from build123d import *

# Parameters (mm, degrees)
SKETCH2_W           = 150
SKETCH2_H           = 75
SKETCH2_W_2         = 25
SKETCH2_H_2         = 62.5
SKETCH2_W_3         = 15
SKETCH2_W_4         = 10
SKETCH2_W_5         = 5
SKETCH2_W_6         = 2.5
SKETCH2_W_7         = 1
BOSS_EXTRUDE1_DEPTH = 20


with BuildPart() as part:
    # Sketch2 → Boss-Extrude1 (new body)
    with BuildSketch(Plane(origin=(0, 0, 0), x_dir=(1, 0, 0), z_dir=(0, 1, 0))):
        with Locations((75, 37.5)):
            Rectangle(SKETCH2_W, SKETCH2_H)
        with Locations((21.5, 36.25)):
            Rectangle(SKETCH2_W_2, SKETCH2_H_2, mode=Mode.SUBTRACT)
        with Locations((66.5, 36.25)):
            Rectangle(SKETCH2_W_3, SKETCH2_H_2, mode=Mode.SUBTRACT)
        with Locations((94, 36.25)):
            Rectangle(SKETCH2_W_4, SKETCH2_H_2, mode=Mode.SUBTRACT)
        with Locations((111.5, 36.25)):
            Rectangle(SKETCH2_W_5, SKETCH2_H_2, mode=Mode.SUBTRACT)
        with Locations((122.75, 36.25)):
            Rectangle(SKETCH2_W_6, SKETCH2_H_2, mode=Mode.SUBTRACT)
        with Locations((127.5, 36.25)):
            Rectangle(SKETCH2_W_7, SKETCH2_H_2, mode=Mode.SUBTRACT)
    extrude(amount=BOSS_EXTRUDE1_DEPTH)


solid = part.part
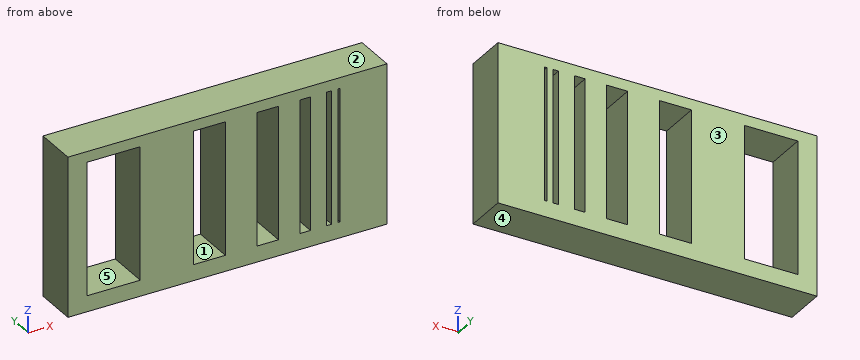
Input: part model. Units: mm. Frame: model coordinates. Face numbers are marked on the shaded views. A direction names the side the tool comes from. Round coordinates to 2 decimals unless told otherwise and drop trailing zeros. Loops run counter-clockwise (first coordinate to the right, second up) from the corner with the lowest first, then second, coordinate; pieces in that order, holes last. Notation, with made-up numbers: (-39, -12) -> (-4, -12) arc R21 ccw to (-4, 23) -> close; hole circle Ø7 at (68.25, 58). An arc over 180 degrees is marked (long way). Answer as a JSON object with one key per item and string values. Group by question number.
1) Section query B-B on y = 17.75. Output: boundary loops of the cut face in (x, z).
2) Draft query along Z for the marked faces 1, 2 and 3. Return one class per face: +Z half, -Z half, draft (parallel to the pull), parting line (faces both ways), or undercut.
3) Reachability of the marked faces 4 and 5 from +Z, -Z, +X, -X, +Y, -Y: full face, straight path, thin tool, end or side. Return the list, or none.
4) Ray query, L1, parallel to Z at x = 73, y = 9.25. Return the intervals inside material, ascending.
5) Section query A-A on z = -12. Output: boundary loops of the cut face in (x, y).
6) Section query C-C on x = 24. Output: boundary loops of the cut face in (y, z), plus the area to 3 significant figures.
Reply:
{
 "1": {"outline": "(0, -75) -> (150, -75) -> (150, 0) -> (0, 0) -> close; hole (9, -67.5) -> (34, -67.5) -> (34, -5) -> (9, -5) -> close; hole (59, -67.5) -> (74, -67.5) -> (74, -5) -> (59, -5) -> close; hole (89, -67.5) -> (99, -67.5) -> (99, -5) -> (89, -5) -> close; hole (109, -67.5) -> (114, -67.5) -> (114, -5) -> (109, -5) -> close; hole (121.5, -67.5) -> (124, -67.5) -> (124, -5) -> (121.5, -5) -> close; hole (127, -67.5) -> (128, -67.5) -> (128, -5) -> (127, -5) -> close"},
 "2": {"face 1": "undercut", "face 2": "+Z half", "face 3": "draft"},
 "3": {"face 4": "-Z, +X, -X, +Y, -Y", "face 5": "+Y, -Y"},
 "4": {"L1": "z = -75 to -67.5, -5 to 0"},
 "5": {"outline": "(0, 0) -> (9, 0) -> (9, 20) -> (0, 20) -> close; (34, 0) -> (59, 0) -> (59, 20) -> (34, 20) -> close; (74, 0) -> (89, 0) -> (89, 20) -> (74, 20) -> close; (99, 0) -> (109, 0) -> (109, 20) -> (99, 20) -> close; (114, 0) -> (121.5, 0) -> (121.5, 20) -> (114, 20) -> close; (124, 0) -> (127, 0) -> (127, 20) -> (124, 20) -> close; (128, 0) -> (150, 0) -> (150, 20) -> (128, 20) -> close"},
 "6": {"outline": "(0, -75) -> (20, -75) -> (20, -67.5) -> (0, -67.5) -> close; (0, -5) -> (20, -5) -> (20, 0) -> (0, 0) -> close", "area": "250 mm2"}
}
